```python
from build123d import *

# Parameters (mm, degrees)
SKETCH1_W               = 50.8
SKETCH1_H               = 25.4
SKETCH1_W_2             = 47.752
SKETCH1_H_2             = 22.352
EXTRUDE_THIN1_DEPTH     = 711.2
CUT_EXTRUDE1_DEPTH      = 714.464252784
CUT_EXTRUDE1_DEPTH_BACK = 714.464252784
SKETCH2_R               = 14.2875


with BuildPart() as part:
    # Sketch1 → Extrude-Thin1 (new body)
    with BuildSketch(Plane(origin=(0, 0, 0), x_dir=(1, 0, 0), z_dir=(0, 1, 0))):
        with Locations((-25.4, -12.7)):
            Rectangle(SKETCH1_W, SKETCH1_H)
        with Locations((-25.4, -12.7)):
            Rectangle(SKETCH1_W_2, SKETCH1_H_2, mode=Mode.SUBTRACT)
    extrude(amount=EXTRUDE_THIN1_DEPTH)

    # Sketch2 → Cut-Extrude1 (cut, two sides: drawn at the far end of the back side and taken through both)
    with BuildSketch(Plane.XY.offset(25.4).offset(-CUT_EXTRUDE1_DEPTH_BACK)):
        with Locations(Location((-25.4, 38.1, 0), (0, 0, 180))):
            Circle(SKETCH2_R)
    extrude(amount=CUT_EXTRUDE1_DEPTH + CUT_EXTRUDE1_DEPTH_BACK, mode=Mode.SUBTRACT)


solid = part.part
```
The model under review builds one solid part; all positions refer to its coordinate system, in mm. A direction names the side the tool comes from. Give positions to 0.01 mm unless a question says otherwise; leave off trailing zeros. Write each loop counter-clockwise with the first axis right and the second up, starting at its lowest first coordinate (ties: lowest second). Pieces come first, ordered by that corner, then holes.
(1) Tool access review of faces 1 (the flat face through (-26, 711.2, 25)), 2 (the flat face through (-26, 351, 23.876)): name each direction out of +Z, -Z, +X, -X, +Y, -Y from which nothing blocks a thin tool from reaching the whole face with its end or side.
(2) Consider section C-C, the plane z = 10.25. Give the boundary of the cut face in (x, y), and give its area (3 significant figures).
(3) Consider section A-A, the plane y = 38.1. Give the boundary of the cut face in (x, z).
(4) The part is to be moulded in two halves that separate along Z. For faces 3 (the cylindrical face through (-11.126, 37.472, 24.627)), 4 (the flat face through (-1.524, 351, 13)), 5 (the flat face through (-26, 351, 25.4)), say which applies: released by +Z, released by -Z, zero draft, split by the parting line, or undercut.
(5) Consider section B-B, the plane x = -25.4. Give the boundary of the cut face in (y, z), and give its area (3 significant figures).
(6) To check wall thickness, follow L1, parallel to Y at x = -25.4, z = 0.4; L2, parallel to Z at x = -36, y = 549.5; L3, parallel to X at y = 666, z = 18. State the ranges of each line that lie inside material, in increasing order.
(7) For P1, Ø4, axis at x = -34, z = 21, coming from the +Y side; P2, Ø3, axis at y = 575.5, z = 8, coming from the +X side, all flat-tipped, find the tip position at first contact; note any pin that passes through.
(8) Consider section D-D, the plane y = 379.5. Give the boundary of the cut face in (x, z), and give its area (3 significant figures).
Returned:
1. face 1: +Z, -Z, +X, -X, +Y
1. face 2: +Y, -Y
2. outline: (-50.8, 0) - (-49.28, 0) - (-49.28, 711.2) - (-50.8, 711.2) - close; (-1.52, 0) - (0, 0) - (0, 711.2) - (-1.52, 711.2) - close
2. area: 2,170 mm2
3. outline: (-50.8, 0) - (-39.69, 0) - (-39.69, 1.52) - (-49.28, 1.52) - (-49.28, 23.88) - (-39.69, 23.88) - (-39.69, 25.4) - (-50.8, 25.4) - close; (-11.11, 0) - (0, 0) - (0, 25.4) - (-11.11, 25.4) - (-11.11, 23.88) - (-1.52, 23.88) - (-1.52, 1.52) - (-11.11, 1.52) - close
4. face 3: zero draft
4. face 4: undercut
4. face 5: released by +Z
5. outline: (0, 0) - (23.81, 0) - (23.81, 1.52) - (0, 1.52) - close; (0, 23.88) - (23.81, 23.88) - (23.81, 25.4) - (0, 25.4) - close; (52.39, 0) - (711.2, 0) - (711.2, 1.52) - (52.39, 1.52) - close; (52.39, 23.88) - (711.2, 23.88) - (711.2, 25.4) - (52.39, 25.4) - close
5. area: 2,080 mm2
6. L1: y = 0 to 23.81, 52.39 to 711.2
6. L2: z = 0 to 1.52, 23.88 to 25.4
6. L3: x = -50.8 to -49.28, -1.52 to 0
7. P1: passes through
7. P2: stops at x = 0
8. outline: (-50.8, 0) - (0, 0) - (0, 25.4) - (-50.8, 25.4) - close; hole (-49.28, 1.52) - (-1.52, 1.52) - (-1.52, 23.88) - (-49.28, 23.88) - close
8. area: 223 mm2
